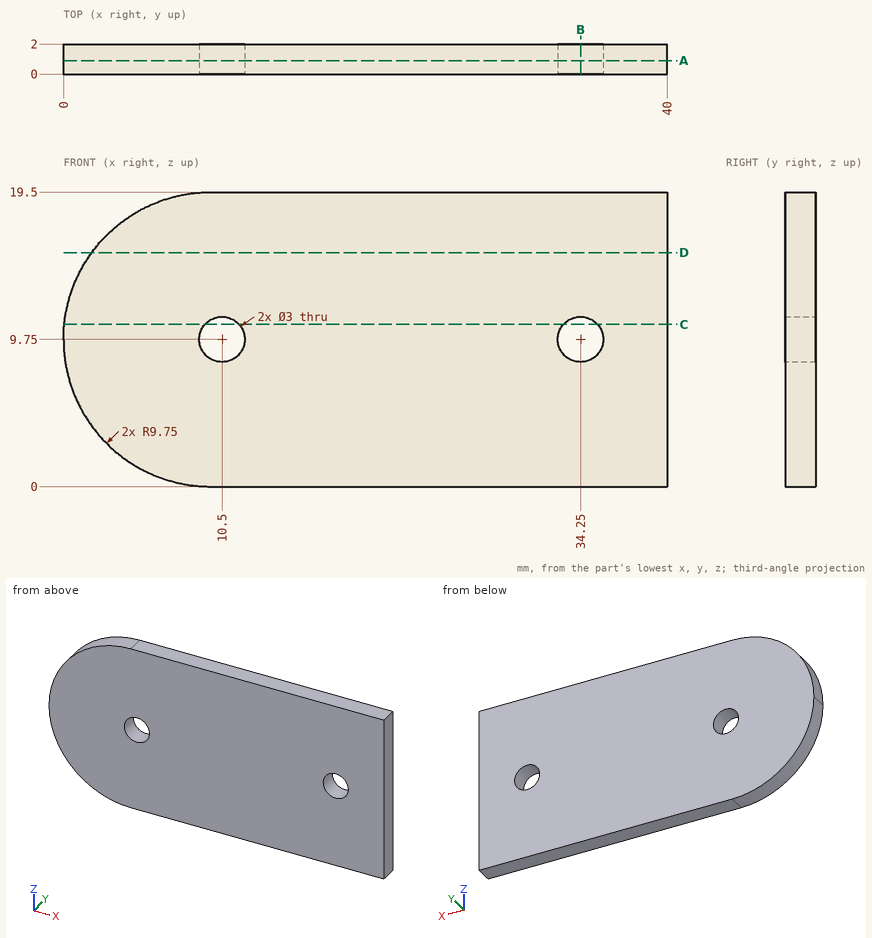
Can you work these out from the drawing? Everything is in mm from the part's minimum corner. Round coordinates to 2 decimals unless told otherwise and drop trailing zeros. Order: outer loops, then holes, each group sorted by start corner. A loop starts at its lowest first (then second) coordinate and runs counter-clockwise, first axis right, second up. Notation, with made-up numbers: M 40.5,-12 L 78.5,-12 A8 ccw 78.5,2 Z; hole C 87,15 d5. An arc over 180 degrees is marked long. One line per question, with ' | ' between items.
1) I want a section at D-D, the plane z = 15.5. Write out the boundary of the cut face in (x, y).
Working result:
outline: M 1.88,0 L 40,0 L 40,2 L 1.88,2 Z
2) I want a section at B-B, the plane x = 34.25. Write out the boundary of the cut face in (y, z).
Working result:
outline: M 0,0 L 2,0 L 2,8.25 L 0,8.25 Z; M 0,11.25 L 2,11.25 L 2,19.5 L 0,19.5 Z
3) I need wall thicknesses on line 1 along X through (y, z) = (0.9, 9.75); line 2 along X through (y, z) = (0.3, 8.5); line 3 along Z through (x, y) = (9.5, 1.15). Which ranges of each line are inside material? Lowest first, please.
Working result:
line 1: 0 to 9, 12 to 32.75, 35.75 to 40 | line 2: 0.08 to 9.67, 11.33 to 33.42, 35.08 to 40 | line 3: 0 to 8.63, 10.87 to 19.5
4) I want a section at A-A, the plane y = 0.9. State how many separate pieces and enclosed holes the cut face has, then the cut area to 3 significant figures.
Working result:
separate pieces: 1 | enclosed holes: 2 | area: 725 mm²
5) For pin 1 Ø5 at (x, z) = (10.5, 9.75) entering from -Y, with a flat end and sliding along its axis, tell me the tip position at first contact or that it passes through.
Working result:
pin 1: y = 0
6) I want a section at C-C, the plane z = 10.75. Write out the boundary of the cut face in (x, y).
Working result:
outline: M 0.05,0 L 9.38,0 L 9.38,2 L 0.05,2 Z; M 11.62,0 L 33.13,0 L 33.13,2 L 11.62,2 Z; M 35.37,0 L 40,0 L 40,2 L 35.37,2 Z
